Check sheet for the modelled part. Datum: model origin and axes. Units: mm. Face numbers are marked on the shaded views. A direction names the side the tool comes from. Round coordinates to 2 decimals unless told otherwise and drop trailing zeros. Write each loop counter-clockwise with the first axis right and the second up, starting at its lowest first coordinate (ties: lowest second). Pieces come first, ordered by that corner, then holes.
Item 1: Release check for a two-part mould opening along Y. For the marked faces 4, 5, 6 and 7 record: pulls with the +Y half, pulls with the -Y half, needs draft (parallel to the pull), parting line crosses it, or undercut.
Item 2: Section check A-A, the plane x = 0. Record the cut outline in (y, z).
Item 3: Material ranges on line 1 along Z through (x, y) = (-2.75, -8.5); line 2 along Y through (x, z) = (2.5, 1); line 3 along X through (y, z) = (3.75, 2.25), recorded low to high.
Item 4: Section check B-B, the plane z = 0.5. Record the cut outline in (x, y).
Item 5: Set-up check for the marked faces 1, 2 and 3: record each of +Z, -Z, +X, -X, +Y, -Y from which the full face is reachable in a straight line by a thin tool's end or side.
Item 6: Depth check by flat-ended pin: pin 1 (1 mm diameter, centred on y = 8.5, z = 3.5, fed in from +X); pin 2 (2 mm diameter, centred on y = -5, z = 4.5, fed in from -X); pin 3 (5 mm diameter, centred on x = -3, y = 5, fed in from +Z); pin 4 (2.5 mm diameter, centred on x = 0, y = 0, fed in from -Z). Enter the tip coordinate at first touch or a pass-through.
Item 7: Section check D-D, the plane y = -6.5. Record the cut outline in (x, z).
Item 8: Section check C-C, the plane z = 7.5. State how many separate pieces and enclosed holes the cut face has, plus the area to 3 significant figures.
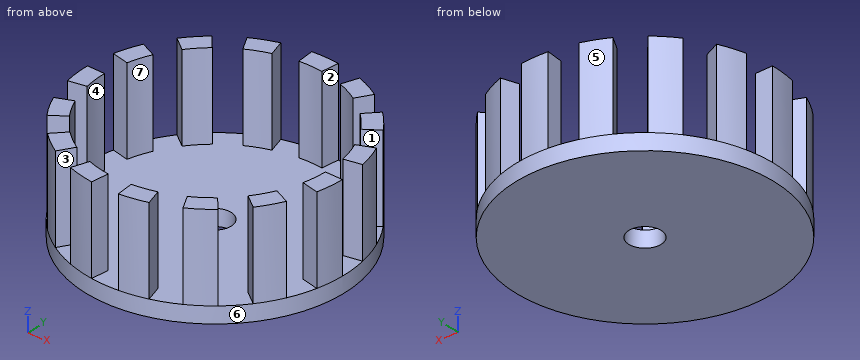
from build123d import *

# Parameters (mm, degrees)
SKETCH_R           = 12
SKETCH_R_2         = 1.5
PAD_DEPTH          = 1.5
PAD001_DEPTH       = 8
POLARPATTERN_COUNT = 15


with BuildPart() as part:
    # Sketch → Pad (new body)
    with BuildSketch(Plane.XY):
        Circle(SKETCH_R)
        Circle(SKETCH_R_2, mode=Mode.SUBTRACT)
    extrude(amount=PAD_DEPTH)

    # Sketch001 → Pad001 (new body)
    with BuildSketch(Plane.XY.offset(1.5)):
        with BuildLine():
            ThreePointArc((1.25, 11.934718), (0, 12), (-1.25, 11.934718))
            Line((-1.25, 11.934718), (-1.082422, 10.334718))
            ThreePointArc((1.082422, 10.334718), (0, 10.391248), (-1.082422, 10.334718))
            Line((1.25, 11.934718), (1.082422, 10.334718))
        make_face()
    pad001 = extrude(amount=PAD001_DEPTH)

    # PolarPattern: Pad001 ×15 about axis
    polarpattern_axis = Axis((0, 0, 1.5), (0, 0, 1))
    for i in range(1, POLARPATTERN_COUNT):
        add(pad001.rotate(polarpattern_axis, i * 360 / POLARPATTERN_COUNT))


solid = part.part
Values found:
1. face 4: undercut
1. face 5: pulls with the +Y half
1. face 6: parting line crosses it
1. face 7: undercut
2. outline: (-12, 0) - (-1.5, 0) - (-1.5, 1.5) - (-12, 1.5) - close; (1.5, 0) - (12, 0) - (12, 9.5) - (10.39, 9.5) - (10.39, 1.5) - (1.5, 1.5) - close
3. line 1: z = 0 to 1.5
3. line 2: y = -11.74 to 11.74
3. line 3: x = -11.4 to -9.69, 9.69 to 11.4
4. outline: circle Ø24 at (0, 0); hole circle Ø3 at (0, 0)
5. face 1: +Z, +X
5. face 2: +Z
5. face 3: +Z, -Y
6. pin 1: stops at x = 8.94
6. pin 2: stops at x = -10.96
6. pin 3: stops at z = 1.5
6. pin 4: passes through
7. outline: (-10.09, 0) - (10.09, 0) - (10.09, 9.5) - (8.95, 9.5) - (8.95, 1.5) - (-8.95, 1.5) - (-8.95, 9.5) - (-10.09, 9.5) - close
8. separate pieces: 15
8. enclosed holes: 0
8. area: 56.4 mm2
